```python
from build123d import *

# Parameters (mm, degrees)
F0_W     = 38
F0_H     = 18
F1_DEPTH = 2.6
F2_R     = 1
F3_DEPTH = 2.6
F4_W     = 6
F4_H     = 8
F5_DEPTH = 3.4
F6_W     = 9
F6_H     = 15
F7_DEPTH = 4


with BuildPart() as f1:
    # F0 (on Top) → F1 (new body)
    with BuildSketch(Plane.XY):
        Rectangle(F0_W, F0_H)
    extrude(amount=F1_DEPTH)

    # F2 (on face) → F3 (cut, through all)
    with BuildSketch(Plane.XY.offset(2.6)):
        with Locations((17, 7)):
            Circle(F2_R)
        with Locations((17, -7)):
            Circle(F2_R)
    extrude(amount=-F3_DEPTH, mode=Mode.SUBTRACT)

    # F4 (on face) → F5 (join)
    with BuildSketch(Plane.XY.offset(2.6)):
        with Locations((16, 0)):
            Rectangle(F4_W, F4_H)
    extrude(amount=F5_DEPTH)

    # F6 (on face) → F7 (join)
    with BuildSketch(Plane.XY.offset(2.6)):
        with Locations((-20.5, 0)):
            Rectangle(F6_W, F6_H)
    extrude(amount=F7_DEPTH)


solid = f1.part
```
Geometry check sheet. Reference: the model listing, model coordinates, mm. A direction names the side the tool comes from. Give positions to 0.01 mm unless a question says otherwise; leave off trailing zeros. Write each loop counter-clockwise with the first axis right and the second up, starting at its lowest first coordinate (ties: lowest second). Pieces come first, ordered by that corner, then holes. Notation, with made-up numbers: (-35, 66.25) - (3, 66.25) arc R19 cw to (3, 85.25) - close; hole circle Ø5 at (-27.75, -36.5). An arc over 180 degrees is marked (long way). Use a Markdown table: item, result.
Q1. Draft check along X on faces 4 (the face through (0, 0, 2.6)), 5 (the face through (-19, 0, 1)), 6 (the face through (16, -4, 4)). Enter one of: pulls with the +X half, pulls with the -X half, needs draft (parallel to the pull), parting line crosses it, or undercut.
Computed:
| item | result |
|---|---|
| face 4 | undercut |
| face 5 | pulls with the -X half |
| face 6 | needs draft |
Q2. Section check D-D, the plane z = 0.5. Enter the section's corners in (x, y), then the cut area to 3 significant figures.
Computed:
| item | result |
|---|---|
| outline | (-19, -9) - (19, -9) - (19, 9) - (-19, 9) - close; hole circle Ø2 at (17, -7); hole circle Ø2 at (17, 7) |
| area | 678 mm² |
Q3. Go/stop test with flat-tipped pins: P1, Ø5.5, axis at x = 6.5, y = 3, coming from the +Z side; P2, Ø1.8, axis at x = -22, y = -0.5, coming from the -Z side; P3, Ø1, axis at x = 16, z = 4, coming from the +Y side; P4, Ø1.6, axis at x = 17, y = 7, coming from the -Z side. Record where each tip stops, or that it passes through.
Computed:
| item | result |
|---|---|
| P1 | stops at z = 2.6 |
| P2 | stops at z = 2.6 |
| P3 | stops at y = 4 |
| P4 | passes through |
Q4. Section check B-B, the plane y = -7. Enter the section's corners in (x, z).
Computed:
| item | result |
|---|---|
| outline | (-25, 2.6) - (-19, 2.6) - (-19, 0) - (16, 0) - (16, 2.6) - (-16, 2.6) - (-16, 6.6) - (-25, 6.6) - close; (18, 0) - (19, 0) - (19, 2.6) - (18, 2.6) - close |
Q5. Section check C-C, the plane x = 17. Enter the section's corners in (y, z).
Computed:
| item | result |
|---|---|
| outline | (-9, 0) - (-8, 0) - (-8, 2.6) - (-9, 2.6) - close; (-6, 0) - (6, 0) - (6, 2.6) - (4, 2.6) - (4, 6) - (-4, 6) - (-4, 2.6) - (-6, 2.6) - close; (8, 0) - (9, 0) - (9, 2.6) - (8, 2.6) - close |
Q6. Thickness scan on L1, parallel to Y at x = 17, z = 1; L2, parallel to X at y = -3.25, z = 4; L3, parallel to Z at x = 5.5, y = 6.75. Record the ranges inside material, lowest first. Write a range as [from, to].
Computed:
| item | result |
|---|---|
| L1 | y = [-9, -8], [-6, 6], [8, 9] |
| L2 | x = [-25, -16], [13, 19] |
| L3 | z = [0, 2.6] |
Q7. Section check A-A, the plane z = 4.75. Enter the section's corners in (x, y), then the cut area to 3 significant figures.
Computed:
| item | result |
|---|---|
| outline | (-25, -7.5) - (-16, -7.5) - (-16, 7.5) - (-25, 7.5) - close; (13, -4) - (19, -4) - (19, 4) - (13, 4) - close |
| area | 183 mm² |
Q8. Set-up check for faces 1 (the face through (-21, 7.5, 5)), 2 (the face through (16, 4, 4)), 3 (the face through (-22, 0, 2.6)): record each of +Z, -Z, +X, -X, +Y, -Y from which the full face is reachable in a straight line by a thin tool's end or side.
Computed:
| item | result |
|---|---|
| face 1 | +Z, +X, -X, +Y |
| face 2 | +Z, +X, +Y |
| face 3 | -Z, -X, +Y, -Y |
